```python
from build123d import *

# Parameters (mm, degrees)
F2_R     = 2.65
F3_DEPTH = 7.101
F5_D     = 5


with BuildPart() as f1:
    # F0 (on Right) → F1 (revolve)
    with BuildSketch(Plane.YZ):
        with BuildLine():
            Line((2.5, 17), (2.5, 102.5))
            Line((2.5, 102.5), (0, 102.5))
            Line((0, 102.5), (0, 111))
            Line((0, 111), (-4.6, 111))
            Line((-4.6, 111), (-4.6, 102))
            Line((-4.6, 102), (-15.294095, 99.134526))
            ThreePointArc((-15.294095, 99.134526), (-17.966767, 97.348704), (-19, 94.304897))
            Line((-19, 94.304897), (-19, 36.5))
            ThreePointArc((-19, 36.5), (-19.43934, 35.43934), (-20.5, 35))
            Line((-20.5, 35), (-23.5, 35))
            ThreePointArc((-23.5, 35), (-24.56066, 34.56066), (-25, 33.5))
            Line((-25, 33.5), (-25, 29.62006))
            ThreePointArc((-25, 29.62006), (-25.525445, 28.26888), (-26.825689, 27.627671))
            Line((-26.825689, 27.627671), (-34, 27))
            Line((-34, 27), (-34, 17))
            Line((-34, 17), (2.5, 17))
        make_face()
    revolve(axis=Axis((0, -26.156189, 0), (0, -1, 0)))

    # F2 (on face) → F3 (cut, through all)
    with BuildSketch(Plane.XZ.offset(4.6)):
        with Locations((-106.25, 0)):
            Circle(F2_R)
        with Locations((-75.130096, -75.130096)):
            Circle(F2_R)
        with Locations((0, -106.25)):
            Circle(F2_R)
        with Locations((75.130096, -75.130096)):
            Circle(F2_R)
        with Locations((106.25, 0)):
            Circle(F2_R)
        with Locations((75.130096, 75.130096)):
            Circle(F2_R)
        with Locations((0, 106.25)):
            Circle(F2_R)
        with Locations((-75.130096, 75.130096)):
            Circle(F2_R)
    extrude(amount=-F3_DEPTH, mode=Mode.SUBTRACT)

    # F5 (through all)
    with Locations(Plane.XZ.offset(34)):
        with Locations((-3.82026, 21.665771), (16.852978, 14.141327), (20.673238, -7.524443), (3.82026, -21.665771), (-16.852978, -14.141327), (-20.673238, 7.524443)):
            Hole(F5_D / 2)


solid = f1.part
```
Can you work these out from the model? Positions are in its coordinate system, mm. A direction names the side the tool comes from. Coordinates: 2 decimals unless noted, no trailing zeros. Loops run counter-clockwise (first coordinate to the right, second up) from the corner with the lowest first, then second, coordinate; pieces in that order, holes last. Notation, with made-up numbers: (68, 10) - (117, 10) arc R8 cw to (117, 17) - close; hole circle Ø8 at (83.5, 25). An arc over 180 degrees is marked (long way). Answer as CSV lines item,"result". Start each with the question number.
1) For pin 1 (5 mm diameter, centred on y = -10, z = -40, fed in from +X); pin 2 (6 mm diameter, centred on x = -75.13, z = 75.13, fed in from -Y); pin 3 (7 mm diameter, centred on x = -106.25, z = 0, fed in from +Y), each with a flat end and sliding along its axis, tell me the tip position at first contact or that it passes through.
2) I need wall thicknesses on line 1 (X direction, y = -6, z = -9.5); line 2 (Y direction, x = -14.5, z = -45); line 3 (Z direction, x = 10, y = -28). Which ranges of each line are inside material? Lowest first, please. Write a range as from..to.
3) Suppose I cut it at A-A (z = -106.25). Please give me the cut outline in (x, y), plus the area to 3 significant figures.
4) Suppose I cut it at B-B (x = 106.25). Please give me the cut outline in (y, z).
5) Thinking about a two-plate mould opening in Y: for faces 4 (the flat face through (32, 0, -98)), 5 (the cylindrical face through (19.52, -15.495, -9.742)), 6 (the conical face through (96.913, -14.775, -21.521)), which applies, pulls with the +Y half, pulls with the -Y half, needs draft (parallel to the pull), parting line crosses it, or undercut?
6) Which directions (+Z, -Z, +X, -X, +Y, -Y) give clear straight access to the entire face, cutting with the end or side of a thin tool? Please do faces 1 (the flat face through (90, -4.6, 49)), 2 (the cylindrical face through (100.063, 1.232, -22.22)), 3 (the flat face through (18, -34, 0)).
Check result:
1,pin 1,"stops at x = 93.53"
1,pin 2,"stops at y = -4.6"
1,pin 3,"stops at y = 0"
2,line 1,"x = -101.18..-14.1, 14.1..19.14, 22.21..101.18"
2,line 2,"y = -19..2.5"
2,line 3,"z = -25.64..-13.75, 13.75..25.64"
3,outline,"(-32.12, -4.6) - (-2.65, -4.6) - (-2.65, 0) - (-32.12, 0) - close; (2.65, -4.6) - (32.12, -4.6) - (32.12, 0) - (2.65, 0) - close"
3,area,"271 mm²"
4,outline,"(-4.6, -32.12) - (0, -32.12) - (0, -2.65) - (-4.6, -2.65) - close; (-4.6, 2.65) - (0, 2.65) - (0, 32.12) - (-4.6, 32.12) - close"
5,face 4,"pulls with the +Y half"
5,face 5,"needs draft"
5,face 6,"pulls with the -Y half"
6,face 1,"-Y"
6,face 2,"+Y"
6,face 3,"+Z, -Z, +X, -X, -Y"
